Input: part model. Units: mm. Frame: model coordinates. A direction names the side the tool comes from. Give positions to 0.01 mm unless a question says otherwise; leave off trailing zeros. Loops run counter-clockwise (first coordinate to the right, second up) from the corner with the lowest first, then second, coordinate; pieces in that order, holes last. Notation, with made-up numbers: M 6.25,32.25 L 18.25,32.25 A11 ccw 18.25,50.25 Z; hole C 65.5,36.25 d7. An arc over 180 degrees is marked long. Use a Markdown table: item, result. Add a question column.
from build123d import *

# Parameters (mm, degrees)
EXTRUDE1_DEPTH = 0.635


with BuildPart() as part:
    # Sketch1 → Extrude1 (new, symmetric)
    with BuildSketch(Plane(origin=(0, 0, 0), x_dir=(1, 0, 0), z_dir=(0, 1, 0))):
        with BuildLine():
            Line((-10.4775, 0), (-7.366, 0))
            ThreePointArc((-7.366, 0), (-7.301957926, 0.969209186), (-7.110945304, 1.921565217))
            ThreePointArc((-7.110945304, 1.921565217), (-6.465513716, 2.804871922), (-5.394551993, 3.02815125))
            ThreePointArc((-5.394551993, 3.02815125), (-4.857704937, 3.086024688), (-4.426323701, 3.410777403))
            ThreePointArc((-4.426323701, 3.410777403), (-0.665227036, 5.54826252), (3.494563676, 4.360478037))
            ThreePointArc((3.494563676, 4.360478037), (3.859883441, 4.17384031), (4.269231255, 4.146885928))
            Line((4.269231255, 4.146885928), (7.740657974, 4.627351162))
            ThreePointArc((7.740657974, 4.627351162), (8.538061077, 5.240237956), (8.417619634, 6.238724705))
            ThreePointArc((8.417619634, 6.238724705), (2.243656673, 10.234452158), (-5.035674849, 9.188034886))
            ThreePointArc((-5.035674849, 9.188034886), (-5.535533941, 8.533256201), (-5.38578247, 7.723213774))
            Line((-5.38578247, 7.723213774), (-4.574680298, 6.538185302))
            ThreePointArc((-4.574680298, 6.538185302), (-4.490147686, 6.185607258), (-4.662218923, 5.866470095))
            Line((-4.662218923, 5.866470095), (-5.056506744, 5.526610046))
            ThreePointArc((-5.056506744, 5.526610046), (-5.294597853, 5.412088501), (-5.558000453, 5.432622154))
            Line((-5.558000453, 5.432622154), (-7.187368065, 6.010571783))
            ThreePointArc((-7.187368065, 6.010571783), (-8.214915896, 6.007492148), (-9.006942583, 5.35284892))
            ThreePointArc((-9.006942583, 5.35284892), (-10.103173936, 2.775586905), (-10.4775, 0))
        make_face()
    extrude(amount=EXTRUDE1_DEPTH, both=True)

    # Mirror1: part across plane


with BuildPart() as part_1:
    add(part.part)
    add(part.part.mirror(Plane(origin=(-10.4775, 0.635, 0), x_dir=(1, 0, 0), z_dir=(0, 0, -1))))


solid = part_1.part
1) Ray query, line 1 (Z direction, x = -5.75, y = -0.45); line 2 (Z direction, x = 4.25, y = 0.3); line 3 (X direction, y = -0.35, z = 4.75). Return the intervals inside material, ascending. Write a range as [from, to].
2) Contact query for a flat-ended pin moving along its axis: P1, Ø6, axis at x = 1.5, z = 1, coming from the +Y side. Output: stop coordinate, or through.
3) Pull-direction query (X, two-part tool) for faces 1 (the cylindrical face through (-5.533, 0.009, -8.545)), 2 (the flat face through (-3, -0.635, 5)), 3 (the flat face through (-6.361, 0.009, 5.718)), 4 (the cylindrical face through (8.532, 0.009, 5.227)); classes: pulls with the +X half, pulls with the -X half, needs draft (parallel to the pull), parting line crosses it, or undercut.
4) Reachability of faces 5 (the cylindrical face through (-0.73, 0.01, -5.54)), 6 (the flat face through (-4.986, 0.009, -7.139)), 7 (the flat face through (5.981, 0.009, 4.384)), 8 (the cylindrical face through (-8.201, 0.009, 6.012)) from +Z, -Z, +X, -X, +Y, -Y: full face, straight path, thin tool, end or side. Return the list, or none.
5) Section query A-A, the plane x = 7.25. Return the cut outline in (y, z) (3 decimals).
6) Section query D-D, the plane z = 8.25. Return the cut outline in (x, y) (3 decimals).
7) Section query B-B, the plane x = -6.5. Return the cut outline in (y, z) (3 decimals), and give its area (3 significant figures).
Entries:
| question | item | result |
|---|---|---|
| 1 | line 1 | z = [-5.5, -3.04], [3.04, 5.5] |
| 1 | line 2 | z = [-9.58, -4.14], [4.14, 9.58] |
| 1 | line 3 | x = [-9.34, -2.94], [2.94, 8.1] |
| 2 | P1 | passes through |
| 3 | face 1 | pulls with the -X half |
| 3 | face 2 | needs draft |
| 3 | face 3 | undercut |
| 3 | face 4 | pulls with the +X half |
| 4 | face 5 | +Y, -Y |
| 4 | face 6 | -X, +Y, -Y |
| 4 | face 7 | +X, +Y, -Y |
| 4 | face 8 | +Z, +Y, -Y |
| 5 | outline | M -0.635,-7.564 L 0.635,-7.564 L 0.635,-4.559 L -0.635,-4.559 Z; M -0.635,4.559 L 0.635,4.559 L 0.635,7.564 L -0.635,7.564 Z |
| 6 | outline | M -5.562,-0.635 L 6.459,-0.635 L 6.459,0.635 L -5.562,0.635 Z |
| 7 | outline | M -0.635,-5.767 L 0.635,-5.767 L 0.635,-2.782 L -0.635,-2.782 Z; M -0.635,2.782 L 0.635,2.782 L 0.635,5.767 L -0.635,5.767 Z |
| 7 | area | 7.58 mm² |
